For this review, take the finished solid that the model builds, in its own axes (mm). Coordinates: 2 decimals unless noted, no trailing zeros. Loops run counter-clockwise (first coordinate to the right, second up) from the corner with the lowest first, then second, coordinate; pieces in that order, holes last.
```python
from build123d import *

# Parameters (mm, degrees)
SKETCH2_W                       = 150
SKETCH2_H                       = 150
BOSS_EXTRUDE2_DEPTH             = 3.175
CHAMFER1_SIZE                   = 25
M3X0_5_TAPPED_HOLE1_D           = 2.5
M3X0_5_TAPPED_HOLE1_CSINK_D     = 3.05
M3X0_5_TAPPED_HOLE1_CSINK_ANGLE = 90


with BuildPart() as part:
    # Sketch2 → Boss-Extrude2 (new body)
    with BuildSketch(Plane(origin=(0, 0, 0), x_dir=(1, 0, 0), z_dir=(0, 1, 0))):
        Rectangle(SKETCH2_W, SKETCH2_H)
    extrude(amount=BOSS_EXTRUDE2_DEPTH)

    # Chamfer1
    chamfer1_edges = [part.edges().sort_by_distance(p)[0] for p in [
        (75, 1.5875, 75),
        (-75, 1.5875, 75),
        (-75, 1.5875, -75),
        (75, 1.5875, -75),
    ]]
    chamfer(chamfer1_edges, length=CHAMFER1_SIZE)

    # M3x0.5 Tapped Hole1 (through all)
    with Locations(Plane(origin=(0, 3.175, 0), x_dir=(1, 0, 0), z_dir=(0, 1, 0))):
        with Locations((-42.5, 35), (42.5, 35), (-42.5, -35), (42.5, -35), (-66.5, 0), (66.5, 0)):
            CounterSinkHole(M3X0_5_TAPPED_HOLE1_D / 2, M3X0_5_TAPPED_HOLE1_CSINK_D / 2, counter_sink_angle=M3X0_5_TAPPED_HOLE1_CSINK_ANGLE)


solid = part.part
```
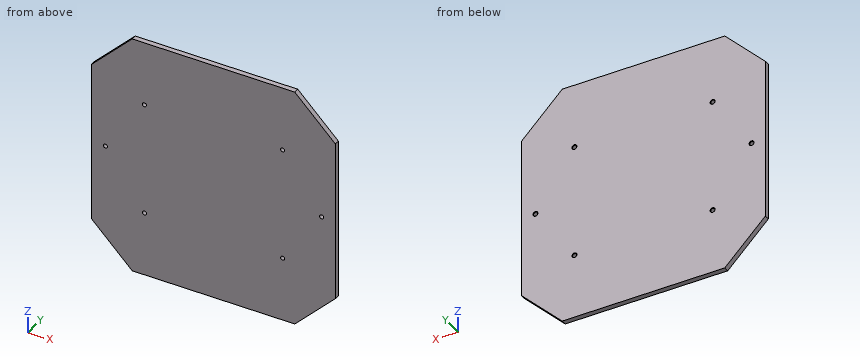
Q1. For pin 1 Ø3 at (x, z) = (-42.5, 35) entering from -Y, flat-tipped, find the tip position at first contact; note if it passes through.
Q2. Consider section C-C (z = -58). State the section outline as (x, y) points (3 decimals).
Q3. Consider section B-B (x = -54). State the section outline as (y, z) points (3 decimals), then the cut area to 3 significant figures.
Q4. Consider section A-A (y = 0.65). State the section outline as (x, z) points.
Q5. Wall thickness on probe 1 along Z at (x, y) = (42.5, 1.1); probe 2 along Z at (x, y) = (-41.5, 0.6); probe 3 along Z at (x, y) = (-67, 0.6): over which ranges is each line inside the solid? List them lowest first.
Model answer:
1. pin 1: stops at y = 0
2. outline: (-67, 0) - (67, 0) - (67, 3.175) - (-67, 3.175) - close
3. outline: (0, -71) - (3.175, -71) - (3.175, 71) - (0, 71) - close
3. area: 451 mm2
4. outline: (-75, -50) - (-50, -75) - (50, -75) - (75, -50) - (75, 50) - (50, 75) - (-50, 75) - (-75, 50) - close; hole circle Ø2.5 at (-66.5, 0); hole circle Ø2.5 at (-42.5, -35); hole circle Ø2.5 at (-42.5, 35); hole circle Ø2.5 at (42.5, -35); hole circle Ø2.5 at (42.5, 35); hole circle Ø2.5 at (66.5, 0)
5. probe 1: z = -75 to -36.25, -33.75 to 33.75, 36.25 to 75
5. probe 2: z = -75 to -35.75, -34.25 to 34.25, 35.75 to 75
5. probe 3: z = -58 to -1.15, 1.15 to 58
